Verification items for this drawing (mm, ordinates from the low corner). A direction names the side the tool comes from. Give positions to 0.01 mm unless a question says otherwise; leave off trailing zeros. Order: outer loops, then holes, each group sorted by start corner. A loop starts at its lowest first (then second) coordinate and runs counter-clockwise, first axis right, second up. Notation, with made-up numbers: M -24.5,-7 L 24.5,-7 A10 ccw 24.5,5 Z; hole C -2,-16.5 d4. An arc over 180 degrees is marked long. Answer as a JSON object with one key per item and string values.
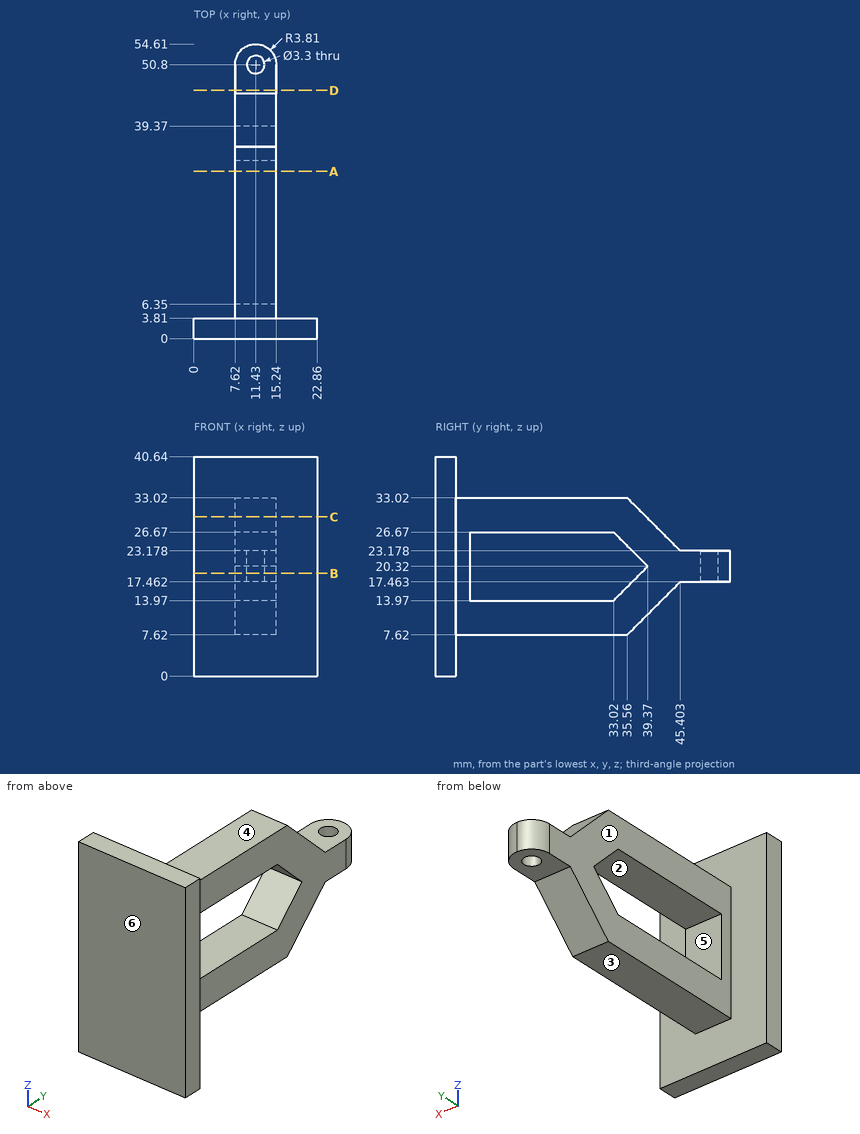
Q1. Tool access check on the marked faces 1, 2 and 3. Record the directions out of +Z, -Z, +X, -X, +Y, -Y that give a thin tool (end or side, any length) a straight path to the whole face; none if there is none.
Resolved:
{"face 1": "+Z, -Z, -X, +Y", "face 2": "+X, -X", "face 3": "-Z, +X, -X, +Y"}
Q2. Gauge pin test, flat ends, axial feed: pin 1 Ø4 at (x, y) = (10.5, 18.5) entering from -Z; pin 2 Ø4 at (x, y) = (9, 26) entering from +Z; pin 3 Ø12 at (y, z) = (17, 21.5) entering from +X. Record the tip position at first contact, or that the pin passes through.
Resolved:
{"pin 1": "stops at z = 7.62", "pin 2": "stops at z = 33.02", "pin 3": "stops at x = 15.24"}
Q3. Section check C-C on z = 29.5. Record the cut outline in (x, y), then the cut area to 3 significant figures.
Resolved:
{"outline": "M 0,0 L 22.86,0 L 22.86,3.81 L 15.24,3.81 L 15.24,39.08 L 7.62,39.08 L 7.62,3.81 L 0,3.81 Z", "area": "356 mm²"}
Q4. Material ranges on L1, parallel to Y at x = 11.43, z = 21.85; L2, parallel to Y at x = 11.43, z = 19.6; L3, parallel to Z at x = 8.75, y = 11.5, recorded low to high.
Resolved:
{"L1": "y = 0 to 6.35, 37.84 to 49.15, 52.45 to 54.61", "L2": "y = 0 to 6.35, 38.65 to 49.15, 52.45 to 54.61", "L3": "z = 7.62 to 13.97, 26.67 to 33.02"}
Q5. Section check B-B on z = 19. Record the cut outline in (x, y).
Resolved:
{"outline": "M 0,0 L 22.86,0 L 22.86,3.81 L 15.24,3.81 L 15.24,6.35 L 7.62,6.35 L 7.62,3.81 L 0,3.81 Z; M 7.62,38.05 L 15.24,38.05 L 15.24,50.8 A3.81 ccw 7.62,50.8 Z; hole C 11.43,50.8 d3.3"}
Q6. Section check D-D on y = 46. Record the cut outline in (x, z).
Resolved:
{"outline": "M 7.62,17.46 L 15.24,17.46 L 15.24,23.18 L 7.62,23.18 Z"}
Q7. Section check A-A on y = 31. Record the cut outline in (x, z).
Resolved:
{"outline": "M 7.62,7.62 L 15.24,7.62 L 15.24,13.97 L 7.62,13.97 Z; M 7.62,26.67 L 15.24,26.67 L 15.24,33.02 L 7.62,33.02 Z"}
Q8. Release check for a two-part mould opening along Y. For the marked faces 4, 5 and 6 record: +Y half, -Y half, draft (parallel to the pull), parting line (faces both ways), or undercut.
Resolved:
{"face 4": "draft", "face 5": "undercut", "face 6": "-Y half"}
